Geometry check sheet. Reference: the model listing, model coordinates, mm. A direction names the side the tool comes from. Give positions to 0.01 mm unless a question says otherwise; leave off trailing zeros. Use a Markdown table: item, result. Add a question column.
1. Material ranges on L1, parallel to Y at x = 1, z = -6; L2, parallel to X at y = 9.5, z = -2.75; L3, parallel to Y at x = -8, z = -0.25 (3 decimals), recorded low to high.
2. Draft check along X on faces 6 (the flat face through (-3.787, -2.159, 3.647)), 7 (the flat face through (3.472, 14.926, -3.352)), 8 (the flat face through (6, 20, 6)), 9 (the flat face through (-3, -10, 3)). Enter one of: pulls with the +X half, pulls with the -X half, needs draft (parallel to the pull), parting line crosses it, or undercut.
3. Depth check by flat-ended pin: P1, Ø1, axis at x = -8.5, y = 14.5, coming from the -Z side; P2, Ø3, axis at x = -0.5, z = 1, coming from the +Y side; P3, Ø4, axis at y = -3.5, z = 1.5, coming from the +X side; P4, Ø2, axis at y = 14.5, z = 1.5, coming from the -X side. Enter the tip coordinate at first touch or a pass-through.
4. Set-up check for faces 1 (the flat face through (3, -10, 3)), 2 (the cylindrical face through (-0.29, 20.29, 2.23)), 3 (the flat face through (3.947, 5.196, -3.807)), 4 (the flat face through (0, -11, 0)), 5 (the flat face through (-3, -10, -3)): record each of +Z, -Z, +X, -X, +Y, -Y from which the full face is reachable in a straight line by a thin tool's end or side.
5. Cross-section at A-A on x = 8. Count the separate pieces of the cut face and the enclosed holes in it, and give its area (3 significant figures).
Autodesk Inventor part; units mm, degrees
ref_plane "작업 평면2" through (0, 0, 0) normal (0, 1, 0) x (-1, 0, 0)
ref_plane "YZ Plane" through (0, 0, 0) normal (1, 0, 0) x (0, 1, 0)
ref_plane "XY Plane" through (0, 0, 0) normal (0, 0, 1) x (1, 0, 0)
sketch "스케치1" plane through (0, 0, 0) normal (0, 1, 0) x (-1, 0, 0)
  line L0 (12, 0) -> (0, -12)
  line L1 (0, -12) -> (-12, 0)
  line L2 (-12, 0) -> (0, 12)
  line L3 (0, 12) -> (12, 0)
  circle A0 centre (0, 0) radius 12 construction
  dimension "d0" = 24
ref_plane "작업 평면1" through (0, 9, 0) normal (0, 1, 0) x (-1, 0, 0)
sketch "스케치2" plane through (0, 9, 0) normal (0, 1, 0) x (-1, 0, 0)
  line L0 (6, 0) -> (0, -6)
  line L1 (0, -6) -> (-6, 0)
  line L2 (-6, 0) -> (0, 6)
  line L3 (0, 6) -> (6, 0)
  circle A0 centre (0, 0) radius 6 construction
  dimension "d2" = 12
loft "로프트1" add profiles "스케치2", "스케치1"
ref_plane "작업 평면2" through (0, 0, 0) normal (0, 1, 0) x (-1, 0, 0)
mirror "미러1" about plane through (0, 9, 0) normal (0, 1, 0) of "로프트1"
mirror "미러2" about plane through (0, 0, 0) normal (0, 1, 0) of "로프트1"
shell "쉘1" thickness 0.5 removed faces 0 ; own thickness 2 on faces at (-5.5, -1.5, -5.5) (5.5, -1.5, 5.5) (-5.5, -1.5, 5.5) (5.5, -1.5, -5.5) (-5.5, 16.5, -5.5) (5.5, 16.5, -5.5) (5.5, 16.5, 5.5) (-5.5, 16.5, 5.5)
sketch "스케치3" plane through (0, -9, -6) normal (0, -1, 0) x (0.7071068, 0, 0.7071068)
  line L0 (0, 8.4853) -> (0, 0)
  line L1 (0, 0) -> (8.4853, 0)
  line L2 (8.4853, 0) -> (8.4853, 8.4853)
  line L3 (8.4853, 8.4853) -> (0, 8.4853)
  point P0 (4.2426, 4.2426)
extrude "돌출1" add sketch "스케치3" along normal blind 2
sketch "스케치4" plane through (-12, 18, 0) normal (0, 1, 0) x (0.7071068, 0, 0.7071068)
  line L0 (0, 0) -> (0, 16.9706)
  line L1 (16.9706, 0) -> (0, 0)
  line L2 (16.9706, 16.9706) -> (16.9706, 0)
  line L3 (0, 16.9706) -> (16.9706, 16.9706)
  point P0 (8.4853, 8.4853)
extrude "돌출2" add sketch "스케치4" along normal blind 5
sketch "스케치5" plane through (-12, 23, 0) normal (0, 1, 0) x (0.7071068, 0, -0.7071068)
  circle A0 centre (8.4853, -8.4853) radius 2.25
  dimension "d14" = 4.5
extrude "돌출3" cut sketch "스케치5" against normal blind 5.5
properties part number "n_4"
Values found:
| question | item | result |
|---|---|---|
| 1 | L1 | y = -7.5 to -2.81, 6.33 to 7.5, 10.5 to 15.19, 17.5 to 23 |
| 1 | L2 | x = -3.58 to -2.13, 2.13 to 3.58 |
| 1 | L3 | y = -5.625 to -0.935, 4.452 to 5.625, 12.375 to 17.065, 17.5 to 23 |
| 2 | face 6 | undercut |
| 2 | face 7 | undercut |
| 2 | face 8 | pulls with the +X half |
| 2 | face 9 | pulls with the -X half |
| 3 | P1 | stops at z = -1.77 |
| 3 | P2 | stops at y = 23 |
| 3 | P3 | stops at x = 10.55 |
| 3 | P4 | stops at x = -9.37 |
| 4 | face 1 | +Z, +X, -Y |
| 4 | face 2 | +Y |
| 4 | face 3 | none |
| 4 | face 4 | +Z, -Z, +X, -X, -Y |
| 4 | face 5 | -Z, -X, -Y |
| 5 | separate pieces | 2 |
| 5 | enclosed holes | 2 |
| 5 | area | 99.0 mm2 |
